Can you work these out from the model? Positions are in its coordinate system, mm. A direction names the side the tool comes from. Coordinates: 2 decimals unless noted, no trailing zeros. Loops run counter-clockwise (first coordinate to the right, second up) from the corner with the lowest first, then second, coordinate; pieces in that order, holes last. Notation, with made-up numbers: (41.25, 0.25) -> (77.25, 0.25) arc R13 ccw to (77.25, 17.25) -> close; hole circle Ø7 at (-28.75, 39.5). An arc over 180 degrees is marked (long way). Use one line per item in the form item = value. Start each with the question number.
(1) Thinking about a two-plate mould opening in Y: for faces 1 (the cylindrical face through (114.89, -75.15, 17.26)), 2 (the flat face through (95, -1, 15)), 3 (the cylindrical face through (90.15, 54.89, 140.14)), 4 (the flat face through (67, -46, 130)), which applies, released by +Y, released by -Y, zero draft, split by the parting line, or undercut?
(2) I'm going to push flat-ended pins straight in: pin 1 (25 mm diameter, centred on x = -103, y = -8, fed in from -Z); pin 2 (12 mm diameter, centred on y = -2.5, z = 55.5, fed in from -X); pin 3 (3 mm diameter, centred on y = -10, z = 91.5, fed in from +X). Where does each tip first touch, or does it pass through?
(3) Imagine slicing it at A-A (x = 18). List the corners of the cut face in (y, z) for me.
(4) Imagine slicing it at D-D (z = 72). List the corners of the cut face in (x, y) for me.
(5) I need wall thicknesses on line 1 (X direction, y = 23.5, z = 28.5); line 2 (Z direction, x = 72, y = 34); line 3 (Y direction, x = 75.5, z = 14). Which ranges of each line are inside material? Lowest first, please. Write a range as [from, to].
(6) Imagine slicing it at B-B (z = 23.5). List the corners of the cut face in (x, y) for me.
(7) On a 3-axis mill with a long thin cutter (end or side, diameter ignored), from which of +Z, -Z, +X, -X, +Y, -Y can I reach the whole of each face in a straight line? I mean faces 5 (the flat face through (-95, -1, 15)), 6 (the flat face through (-73, -52, 35)), 7 (the flat face through (89, 25, 83)), 8 (the cylindrical face through (-90.15, -54.89, 140.14)). Say none if no direction works.
(8) Imagine slicing it at C-C (y = 0.5). List the corners of the cut face in (x, z) for me, plus the area to 3 significant figures.
```python
from build123d import *

# Parameters (mm, degrees)
PAD_DEPTH            = 35
PAD001_DEPTH         = 20
SKETCH002_W          = 140
SKETCH002_H          = 80
POCKET_DEPTH         = 150.001
PAD002_DEPTH         = 25
PAD003_DEPTH         = 25
SKETCH006_W          = 140
SKETCH006_H          = 15
POCKET001_DEPTH      = 80.001
POCKET001_DEPTH_BACK = -80.001
SKETCH007_W          = 80
SKETCH007_H          = 15
POCKET002_DEPTH      = 120.001
POCKET002_DEPTH_BACK = -120.001


with BuildPart() as part:
    # Sketch (on XY_Plane of Origin) → Pad (new body)
    with BuildSketch(Plane.XY):
        with BuildLine():
            Line((-120, 63), (-120, -63))
            ThreePointArc((-120, -63), (-115.020815, -75.020815), (-103, -80))
            Line((-103, -80), (103, -80))
            ThreePointArc((103, -80), (115.020815, -75.020815), (120, -63))
            Line((120, -63), (120, 63))
            ThreePointArc((120, 63), (115.020815, 75.020815), (103, 80))
            Line((103, 80), (-103, 80))
            ThreePointArc((-103, 80), (-115.020815, 75.020815), (-120, 63))
        make_face()
    extrude(amount=PAD_DEPTH)

    # Sketch001 (on XY_Plane of Origin) → Pad001 (join)
    with BuildSketch(Plane.XY.offset(150)):
        with BuildLine():
            Line((-95, 43), (-95, -43))
            ThreePointArc((-95, -43), (-90.020815, -55.020815), (-78, -60))
            Line((-78, -60), (78, -60))
            ThreePointArc((78, -60), (90.020815, -55.020815), (95, -43))
            Line((95, -43), (95, 43))
            ThreePointArc((95, 43), (90.020815, 55.020815), (78, 60))
            Line((78, 60), (-78, 60))
            ThreePointArc((-78, 60), (-90.020815, 55.020815), (-95, 43))
        make_face()
    extrude(amount=-PAD001_DEPTH)

    # Sketch002 (on Face19 of Pad001) → Pocket (cut, through all)
    with BuildSketch(Plane.XY.offset(150)):
        Rectangle(SKETCH002_W, SKETCH002_H)
    extrude(amount=-POCKET_DEPTH, mode=Mode.SUBTRACT)

    # Sketch003 (on YZ_Plane of Origin) → Pad002 (join, symmetric)
    with BuildSketch(Plane.YZ):
        Polygon((-60, 130), (-80, 35), (-40, 35), (-40, 130), align=None)
    pad002 = extrude(amount=PAD002_DEPTH, both=True)

    # Mirrored: Pad002 across Sketch003 V_Axis
    add(pad002.mirror(Plane(origin=(0, 0, 0), x_dir=(1, 0, 0), z_dir=(0, 1, 0))))

    # Sketch005 (on XZ_Plane of Origin) → Pad003 (join, symmetric)
    with BuildSketch(Plane.XZ):
        Polygon((-70, 130), (-70, 35), (-120, 35), (-95, 130), align=None)
    pad003 = extrude(amount=PAD003_DEPTH, both=True)

    # Mirrored001: Pad003 across Sketch005 V_Axis
    add(pad003.mirror(Plane(origin=(0, 0, 0), x_dir=(0, -1, 0), z_dir=(1, 0, 0))))

    # Sketch006 (on XZ_Plane of Origin) → Pocket001 (cut, two sides)
    with BuildSketch(Plane.XZ) as pocket001_sk:
        with Locations((0, 7.5)):
            Rectangle(SKETCH006_W, SKETCH006_H)
    extrude(amount=-POCKET001_DEPTH, mode=Mode.SUBTRACT)
    extrude(pocket001_sk.sketch, amount=-POCKET001_DEPTH_BACK, mode=Mode.SUBTRACT)

    # Sketch007 (on YZ_Plane of Origin) → Pocket002 (cut, two sides)
    with BuildSketch(Plane.YZ) as pocket002_sk:
        with Locations((0, 7.5)):
            Rectangle(SKETCH007_W, SKETCH007_H)
    extrude(amount=-POCKET002_DEPTH, mode=Mode.SUBTRACT)
    extrude(pocket002_sk.sketch, amount=-POCKET002_DEPTH_BACK, mode=Mode.SUBTRACT)


solid = part.part
```
Worked out:
q1.face_1 = released by -Y
q1.face_2 = undercut
q1.face_3 = released by +Y
q1.face_4 = zero draft
q2.pin_1 = 15
q2.pin_2 = -116.18
q2.pin_3 = 105.53
q3.outline = (-80, 15) -> (-40, 15) -> (-40, 150) -> (-60, 150) -> (-60, 130) -> (-80, 35) -> close; (40, 15) -> (80, 15) -> (80, 35) -> (60, 130) -> (60, 150) -> (40, 150) -> close
q4.outline = (-110.26, -25) -> (-70, -25) -> (-70, 25) -> (-110.26, 25) -> close; (-25, -72.21) -> (25, -72.21) -> (25, -40) -> (-25, -40) -> close; (-25, 40) -> (25, 40) -> (25, 72.21) -> (-25, 72.21) -> close; (70, -25) -> (110.26, -25) -> (110.26, 25) -> (70, 25) -> close
q5.line_1 = [-120, -70], [70, 120]
q5.line_2 = [15, 35], [130, 150]
q5.line_3 = [-80, -40], [40, 80]
q6.outline = (-120, -63) arc R17 ccw to (-103, -80) -> (103, -80) arc R17 ccw to (120, -63) -> (120, 63) arc R17 ccw to (103, 80) -> (-103, 80) arc R17 ccw to (-120, 63) -> close; hole (-70, -40) -> (70, -40) -> (70, 40) -> (-70, 40) -> close
q7.face_5 = -Z, +X, -X
q7.face_6 = -X, -Y
q7.face_7 = +X, -X, +Y
q7.face_8 = +Z, -X, -Y
q8.outline = (-120, 15) -> (-70, 15) -> (-70, 150) -> (-95, 150) -> (-95, 130) -> (-120, 35) -> close; (70, 15) -> (120, 15) -> (120, 35) -> (95, 130) -> (95, 150) -> (70, 150) -> close
q8.area = 10,100 mm2
